from build123d import *

# Parameters (mm, degrees)
EXTRUDE_1_DEPTH     = 60
SKETCH_2_R          = 3
CUT_EXTRUDE_1_DEPTH = 69.007352544
SKETCH_3_R          = 3
CUT_EXTRUDE_2_DEPTH = 69.007352544


with BuildPart() as part:
    # 草图1 → 凸台-拉伸1 (new body)
    with BuildSketch(Plane.XY):
        Polygon((0, 0), (5, 0), (5, -20), (25, -20), (25, -25), (0, -25), align=None)
    extrude(amount=EXTRUDE_1_DEPTH)

    # 草图2 → 切除-拉伸1 (cut, through all)
    with BuildSketch(Plane(origin=(0, -20, 0), x_dir=(1, 0, 0), z_dir=(0, 1, 0))):
        with Locations(Location((15, -6, 0), (0, 0, 180))):
            Circle(SKETCH_2_R)
        with Locations(Location((15, -52, 0), (0, 0, 180))):
            Circle(SKETCH_2_R)
    extrude(amount=-CUT_EXTRUDE_1_DEPTH, mode=Mode.SUBTRACT)

    # 草图3 → 切除-拉伸2 (cut, through all)
    with BuildSketch(Plane(origin=(5, 0, 0), x_dir=(0, 0, -1), z_dir=(1, 0, 0))):
        with Locations(Location((-6, -10, 0), (0, 0, 90))):
            Circle(SKETCH_3_R)
        with Locations(Location((-52, -10, 0), (0, 0, 90))):
            Circle(SKETCH_3_R)
    extrude(amount=-CUT_EXTRUDE_2_DEPTH, mode=Mode.SUBTRACT)


solid = part.part
The listing builds one solid part. Answer for the finished solid, in the listing's coordinates (mm). A direction names the side the tool comes from. Round coordinates to 2 decimals unless told otherwise and drop trailing zeros. Order: outer loops, then holes, each group sorted by start corner. A loop starts at its lowest first (then second) coordinate and runs counter-clockwise, first axis right, second up. Notation, with made-up numbers: (44.5, 28) -> (82.5, 28) arc R19 cw to (82.5, 40) -> close; hole circle Ø5 at (54, 47). An arc over 180 degrees is marked (long way). Write each question's results on one line, items separated by ' | '. Start each with the question number.
Q1. The mould has two halves that part along Y. Classify faces 1 (the flat face through (13, -25, 30)), 2 (the flat face through (2, 0, 30)), 3 (the flat face through (5, -10, 30)), 4 (the cylindrical face through (2.5, -12.4, 4.2)): pulls with the +Y half, pulls with the -Y half, needs draft (parallel to the pull), parting line crosses it, or undercut.
Q2. Which of the six approach directions +Z, -Z, +X, -X, +Y, -Y give full straight-line access (tool end or side, diameter ignored) to faces 5 (the flat face through (15, -20, 30)), 6 (the flat face through (4, -18, 0))?
Q3. Straight lines are drawn through the part: probe 1 along Z at (x, y) = (15, -23.5); probe 2 along X at (y, z) = (-6.5, 17); probe 3 along Y at (x, z) = (20.5, 13). For each, find the intervals that lie inside material, in ascending order. Write a range as from..to.
Q4. Find section B-B (z = 6). Determine the outline of the cut face in (x, y), then the cut area to 3 significant figures.
Q5. Each of these flat-tipped pins is pushed along its axis until it touches: pin 1 (8 mm diameter, centred on y = -10, z = 6, fed in from +X); pin 2 (6 mm diameter, centred on x = 9, z = 22.5, fed in from +Y). Where does it stop, or does it pass through?
Q6. Find section A-A (y = -10). Determine the outline of the cut face in (x, z), then the cut area to 3 significant figures.
Q7. Find section C-C (x = 16.75). Determine the outline of the cut face in (y, z), then the cut area to 3 significant figures.
Q8. Find section D-D (x = 3). Determine the outline of the cut face in (y, z), then the cut area to 3 significant figures.
Worked answers:
1) face 1: pulls with the -Y half | face 2: pulls with the +Y half | face 3: needs draft | face 4: undercut
2) face 5: +Z, -Z, +X, +Y | face 6: -Z, +X, -X, +Y, -Y
3) probe 1: z = 0..3, 9..49, 55..60 | probe 2: x = 0..5 | probe 3: y = -25..-20
4) outline: (0, -25) -> (12, -25) -> (12, -20) -> (5, -20) -> (5, -13) -> (0, -13) -> close; (0, -7) -> (5, -7) -> (5, 0) -> (0, 0) -> close; (18, -25) -> (25, -25) -> (25, -20) -> (18, -20) -> close | area: 165 mm2
5) pin 1: stops at x = 5 | pin 2: stops at y = -20
6) outline: (0, 0) -> (5, 0) -> (5, 3) -> (0, 3) -> close; (0, 9) -> (5, 9) -> (5, 49) -> (0, 49) -> close; (0, 55) -> (5, 55) -> (5, 60) -> (0, 60) -> close | area: 240 mm2
7) outline: (-25, 0) -> (-20, 0) -> (-20, 3.56) -> (-25, 3.56) -> close; (-25, 8.44) -> (-20, 8.44) -> (-20, 49.56) -> (-25, 49.56) -> close; (-25, 54.44) -> (-20, 54.44) -> (-20, 60) -> (-25, 60) -> close | area: 251 mm2
8) outline: (-25, 0) -> (0, 0) -> (0, 60) -> (-25, 60) -> close; hole circle Ø6 at (-10, 6); hole circle Ø6 at (-10, 52) | area: 1,440 mm2
